The listing builds one solid part. Answer for the finished solid, in the listing's coordinates (mm). A direction names the side the tool comes from. Round coordinates to 2 decimals unless told otherwise and drop trailing zeros. Order: outer loops, then holes, each group sorted by start corner. A loop starts at its lowest first (then second) coordinate and runs counter-clockwise, first axis right, second up. Notation, with made-up numbers: (0.25, -29.75) - (48.25, -29.75) arc R24 ccw to (48.25, 5.25) - close; hole circle Ø7 at (9, 9.5). An arc over 180 degrees is marked (long way). Write item = value, one per line.
from build123d import *

# Parameters (mm, degrees)
F0_W         = 50
F0_H         = 15
F0_R         = 2
F1_DEPTH     = 10
F2_R         = 3.6792614691
F3_T1_DEPTH  = 20.2290713461
F3_T4_ANGLE  = 90
F3_T6_ANGLE  = 90
F3_T8_ANGLE  = 90
F3_T10_ANGLE = 90
F4_D         = 4.5
F4_DEPTH     = 0.5
F4_TIP       = 1.3519363928
F5_DEPTH     = 7


# Not quite as in the source:
# - a fillet or chamfer that OpenCascade refuses, or shapes differently, is made with other operations: its cross-section is extruded or revolved along the edge and cut away or added


with BuildPart() as f1:
    # F0 (on Top) → F1 (new body)
    with BuildSketch(Plane.XY):
        Rectangle(F0_W, F0_H)
        with Locations((-12.5, 0)):
            Circle(F0_R, mode=Mode.SUBTRACT)
        with Locations((12.5, 0)):
            Circle(F0_R, mode=Mode.SUBTRACT)
        with Locations((12.5, 0)):
            Circle(F0_R)
        with Locations((-12.5, 0)):
            Circle(F0_R)
    extrude(amount=F1_DEPTH)

    # F2
    f2_edges = [f1.edges().sort_by_distance(p)[0] for p in [
        (0, -7.5, 10),
        (-25, 0, 10),
        (25, 0, 10),
        (0, 7.5, 10),
    ]]
    fillet(f2_edges, radius=F2_R)

    # F3: fillet of radius 4.0916285384 on 4 edges, made by hand

    # F3_s2 → F3_t1 (cut)
    with BuildSketch(Plane.XY.offset(-10.2290713461)):
        with BuildLine():
            ThreePointArc((-20.9083714616, 7.5), (-23.8015897472, 6.3015897472), (-25, 3.4083714616))
            Line((-25, 3.4083714616), (-25, 7.5))
            Line((-25, 7.5), (-20.9083714616, 7.5))
        make_face()
        with BuildLine():
            ThreePointArc((-20.9083714616, -7.5), (-23.8015897472, -6.3015897472), (-25, -3.4083714616))
            Line((-25, -3.4083714616), (-25, -7.5))
            Line((-25, -7.5), (-20.9083714616, -7.5))
        make_face()
        with BuildLine():
            ThreePointArc((25, 3.4083714616), (23.8015897472, 6.3015897472), (20.9083714616, 7.5))
            Line((20.9083714616, 7.5), (25, 7.5))
            Line((25, 7.5), (25, 3.4083714616))
        make_face()
        with BuildLine():
            ThreePointArc((25, -3.4083714616), (23.8015897472, -6.3015897472), (20.9083714616, -7.5))
            Line((20.9083714616, -7.5), (25, -7.5))
            Line((25, -7.5), (25, -3.4083714616))
        make_face()
    extrude(amount=F3_T1_DEPTH, mode=Mode.SUBTRACT)

    # F3_s3 → F3_t4 (revolve, cut)
    with BuildSketch(Plane.YZ.offset(20.9083714616)):
        with BuildLine():
            ThreePointArc((-3.8207385309, 10), (-6.4223692655, 8.9223692655), (-7.5, 6.3207385309))
            Line((-7.5, 6.3207385309), (-7.5, 10))
            Line((-7.5, 10), (-3.8207385309, 10))
        make_face()
    revolve(axis=Axis((20.9083714616, -3.4083714616, 10), (0, 0, 1)), revolution_arc=F3_T4_ANGLE, mode=Mode.SUBTRACT)

    # F3_s5 → F3_t6 (revolve, cut)
    with BuildSketch(Plane.XZ.offset(-3.4083714616)):
        with BuildLine():
            ThreePointArc((21.3207385309, 10), (23.9223692655, 8.9223692655), (25, 6.3207385309))
            Line((25, 6.3207385309), (25, 10))
            Line((25, 10), (21.3207385309, 10))
        make_face()
    revolve(axis=Axis((20.9083714616, 3.4083714616, 10), (0, 0, 1)), revolution_arc=F3_T6_ANGLE, mode=Mode.SUBTRACT)

    # F3_s7 → F3_t8 (revolve, cut)
    with BuildSketch(Plane.XZ.offset(3.4083714616)):
        with BuildLine():
            ThreePointArc((-21.3207385309, 10), (-23.9223692655, 8.9223692655), (-25, 6.3207385309))
            Line((-25, 6.3207385309), (-25, 10))
            Line((-25, 10), (-21.3207385309, 10))
        make_face()
    revolve(axis=Axis((-20.9083714616, -3.4083714616, 10), (0, 0, 1)), revolution_arc=F3_T8_ANGLE, mode=Mode.SUBTRACT)

    # F3_s9 → F3_t10 (revolve, cut)
    with BuildSketch(Plane.YZ.offset(-20.9083714616)):
        with BuildLine():
            ThreePointArc((3.8207385309, 10), (6.4223692655, 8.9223692655), (7.5, 6.3207385309))
            Line((7.5, 6.3207385309), (7.5, 10))
            Line((7.5, 10), (3.8207385309, 10))
        make_face()
    revolve(axis=Axis((-20.9083714616, 3.4083714616, 10), (0, 0, 1)), revolution_arc=F3_T10_ANGLE, mode=Mode.SUBTRACT)

    # F4
    with Locations(Plane(origin=(0, 0, 0), x_dir=(1, 0, 0), z_dir=(0, 0, -1))):
        with Locations((0, 0)):
            Hole(F4_D / 2, depth=F4_DEPTH)
            with Locations((0, 0, -(F4_DEPTH + F4_TIP / 2))):  # 118° drill point
                Cone(0, F4_D / 2, F4_TIP, mode=Mode.SUBTRACT)

    # F0 (on Top) → F5 (join)
    with BuildSketch(Plane.XY):
        with Locations((12.5, 0)):
            Circle(F0_R)
        with Locations((-12.5, 0)):
            Circle(F0_R)
    extrude(amount=-F5_DEPTH)


solid = f1.part
Q1. Determine the mould class of faces 3 (the face through (-13, 0, -7)), 4 (the face through (-23.77, 6.333, 3.116)), 5 (the face through (0, 3, 0)) for opening direction X: released by +X, released by -X, zero draft, split by the parting line, or undercut.
Model answer:
face_3 = zero draft
face_4 = released by -X
face_5 = undercut
Q2. Flat-ended cylindrical pins translate along their axes: P1, Ø3, axis at x = 3.5, y = -3, coming from the -Z side; P2, Ø3.5, axis at x = 0, y = 0, coming from the -Z side; P3, Ø1, axis at y = 0, z = 7.5, coming from the -X side. Find the tip coordinate at first contact, or state that the pin passes through.
Model answer:
P1 = 0
P2 = 0.8
P3 = -24.94
Q3. Section B-B on x = 12.5 is taken. Determine the outline of the cut face in (y, z), then the cut area to 3 significant figures.
Model answer:
outline = (-7.5, 0) - (-2, 0) - (-2, -7) - (2, -7) - (2, 0) - (7.5, 0) - (7.5, 6.32) arc R3.68 ccw to (3.82, 10) - (-3.82, 10) arc R3.68 ccw to (-7.5, 6.32) - close
area = 172 mm^2
Q4. Section A-A on z = 3 is taken. Determine the outline of the cut face in (x, y), then the cut area to 3 significant figures.
Model answer:
outline = (-25, -3.41) arc R4.09 ccw to (-20.91, -7.5) - (20.91, -7.5) arc R4.09 ccw to (25, -3.41) - (25, 3.41) arc R4.09 ccw to (20.91, 7.5) - (-20.91, 7.5) arc R4.09 ccw to (-25, 3.41) - close
area = 736 mm^2
Q5. Find the intervals of material crossed by line 1 (Y direction, x = 0, z = 0.3); line 2 (Z direction, x = 17.5, y = 1); line 3 (X direction, y = 1, z = -2), in increasing order. Write a range as from..to.
Model answer:
line_1 = -7.5..-2.25, 2.25..7.5
line_2 = 0..10
line_3 = -14.23..-10.77, 10.77..14.23
Q6. For faces 1 (the face through (-14.1, -1.2, -3.5)), 2 (the face through (0, 0, 10)), determine the directions among +Z, -Z, +X, -X, +Y, -Y from which every point of the face is accessible in a straight line to the end or side of a thin tool.
Model answer:
face_1 = -Z
face_2 = +Z, +X, -X, +Y, -Y
